Geometry check sheet. Reference: the model listing, model coordinates, mm. Face numbers are marked on the shaded views. Round coordinates to 2 decimals unless told otherwise and drop trailing zeros. Write each loop counter-clockwise with the first axis right and the second up, starting at its lowest first coordinate (ties: lowest second). Pieces come first, ordered by that corner, then holes. Notation, with made-up numbers: M 28.25,14 L 67.25,14 A19 ccw 67.25,32 Z; hole C 30,60.25 d6. An arc over 180 degrees is marked long. Answer in a Markdown table with one row per item. Add a question column.
from build123d import *

# Parameters (mm, degrees)
SKETCH_1_R      = 21
SKETCH_1_R_2    = 1.75
SKETCH_1_W      = 40.5
SKETCH_1_H      = 20.2
EXTRUDE_1_DEPTH = 5


with BuildPart() as part:
    # 草图1 → 凸台-拉伸1 (new body)
    with BuildSketch(Plane.XY):
        with BuildLine():
            Line((106.5, -30), (-106.5, -30))
            ThreePointArc((-106.5, -30), (-110.035533906, -28.535533906), (-111.5, -25))
            Line((-111.5, -25), (-111.5, 25))
            ThreePointArc((-111.5, 25), (-110.035533906, 28.535533906), (-106.5, 30))
            Line((-106.5, 30), (106.5, 30))
            ThreePointArc((106.5, 30), (110.035533906, 28.535533906), (111.5, 25))
            Line((111.5, 25), (111.5, -25))
            ThreePointArc((111.5, -25), (110.035533906, -28.535533906), (106.5, -30))
        make_face()
        with Locations((-80, 0)):
            Circle(SKETCH_1_R, mode=Mode.SUBTRACT)
        with Locations((80, 0)):
            Circle(SKETCH_1_R, mode=Mode.SUBTRACT)
        with Locations((33.788860906, -4.762314657)):
            Circle(SKETCH_1_R_2, mode=Mode.SUBTRACT)
        with Locations((33.788860906, 5.237685343)):
            Circle(SKETCH_1_R_2, mode=Mode.SUBTRACT)
        with Locations((-14.211139094, -4.762314657)):
            Circle(SKETCH_1_R_2, mode=Mode.SUBTRACT)
        with Locations((-14.211139094, 5.237685343)):
            Circle(SKETCH_1_R_2, mode=Mode.SUBTRACT)
        with Locations((-54.5, -17.5)):
            Circle(SKETCH_1_R_2, mode=Mode.SUBTRACT)
        with Locations((-105.5, -17.5)):
            Circle(SKETCH_1_R_2, mode=Mode.SUBTRACT)
        with Locations((-105.5, 17.5)):
            Circle(SKETCH_1_R_2, mode=Mode.SUBTRACT)
        with Locations((-54.5, 17.5)):
            Circle(SKETCH_1_R_2, mode=Mode.SUBTRACT)
        with Locations((54.5, -17.5)):
            Circle(SKETCH_1_R_2, mode=Mode.SUBTRACT)
        with Locations((54.5, 17.5)):
            Circle(SKETCH_1_R_2, mode=Mode.SUBTRACT)
        with Locations((105.5, -17.5)):
            Circle(SKETCH_1_R_2, mode=Mode.SUBTRACT)
        with Locations((105.5, 17.5)):
            Circle(SKETCH_1_R_2, mode=Mode.SUBTRACT)
        with Locations((9.788860906, 0.237685343)):
            Rectangle(SKETCH_1_W, SKETCH_1_H, mode=Mode.SUBTRACT)
    extrude(amount=EXTRUDE_1_DEPTH)


solid = part.part
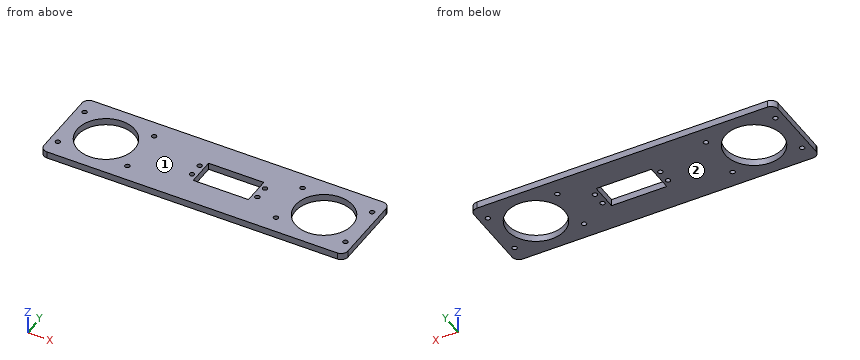
Item 1: Mould release check, pull along Z, two halves, no side actions. Record for the marked faces 1 and 2: +Z half, -Z half, draft (parallel to the pull), parting line (faces both ways), or undercut.
Item 2: Gauge pin test, flat end, axial feed: pin 1 Ø5.5 at (x, y) = (105.5, -17.5) entering from +Z. Record the tip position at first contact, or that the pin passes through.
Item 3: Section check B-B, the plane x = 80. Record the boundary of the cut face in (y, z), and give its area (3 significant figures).
Item 4: Section check A-A, the plane y = 0. Record the boundary of the cut face in (x, z).
Item 5: Section check C-C, the plane z = 3.9. Give the number of separate pieces and of enclosed holes in the cut face, and give its area (3 significant figures).
Item 6: Scan lines: probe 1 along Y at (x, z) = (54.5, 2.1); probe 2 along Y at (x, z) = (29, 0.4); probe 3 along X at (y, z) = (-1, 3.9). Record each from-to range of solid material in increasing order. Write a range as from..to.
Result sheet:
| question | item | result |
|---|---|---|
| 1 | face 1 | +Z half |
| 1 | face 2 | -Z half |
| 2 | pin 1 | stops at z = 5 |
| 3 | outline | M -30,0 L -21,0 L -21,5 L -30,5 Z; M 21,0 L 30,0 L 30,5 L 21,5 Z |
| 3 | area | 90.0 mm^2 |
| 4 | outline | M -111.5,0 L -101,0 L -101,5 L -111.5,5 Z; M -59,0 L -10.46,0 L -10.46,5 L -59,5 Z; M 30.04,0 L 59,0 L 59,5 L 30.04,5 Z; M 101,0 L 111.5,0 L 111.5,5 L 101,5 Z |
| 5 | separate pieces | 1 |
| 5 | enclosed holes | 15 |
| 5 | area | 9,650 mm^2 |
| 6 | probe 1 | y = -30..-19.25, -15.75..15.75, 19.25..30 |
| 6 | probe 2 | y = -30..-9.86, 10.34..30 |
| 6 | probe 3 | x = -111.5..-100.98, -59.02..-10.46, 30.04..59.02, 100.98..111.5 |
